```python
from build123d import *

# Parameters (mm, degrees)
SKETCH_1_R          = 12.5
SKETCH_1_R_2        = 10
EXTRUDE_1_DEPTH     = 120
SKETCH_2_R          = 3.5
CUT_EXTRUDE_1_DEPTH = 12.5
SWEEP_3_PROFILE_R   = 3.5


with BuildPart() as part:
    # 草图1 → 凸台-拉伸1 (new body)
    with BuildSketch(Plane(origin=(0, 0, 0), x_dir=(1, 0, 0), z_dir=(0, 1, 0))):
        Circle(SKETCH_1_R)
        Circle(SKETCH_1_R_2, mode=Mode.SUBTRACT)
    extrude(amount=EXTRUDE_1_DEPTH)

    # 草图2 → 切除-拉伸1 (cut, symmetric)
    with BuildSketch(Plane(origin=(0, 0, 0), x_dir=(0, 0, -1), z_dir=(1, 0, 0))):
        with Locations((0, 60)):
            Circle(SKETCH_2_R)
    extrude(amount=CUT_EXTRUDE_1_DEPTH, both=True, mode=Mode.SUBTRACT)

    # 切除-扫描3: sweep along a path in 草图10
    with BuildLine(Plane(origin=(0, 0, 0), x_dir=(0.342020143, 0, -0.939692621), z_dir=(0.939692621, 0, 0.342020143))) as sweep_3_path:
        Line((42.494333557, 116.01263537), (-37.5, 60))
        Line((-37.5, 60), (79.181849156, -21.701510351))
    # 切除-扫描3 profile (on start of the path) → 切除-扫描3 (sweep, cut)
    with BuildSketch(Plane(origin=(14.533918054, 116.01263537, -39.931611668), x_dir=(0, 0.801864671, 0.59750569), z_dir=(-0.2801665, -0.573576436, 0.769751131))):
        Circle(SWEEP_3_PROFILE_R)
    sweep(path=sweep_3_path.line, transition=Transition.RIGHT, mode=Mode.SUBTRACT)


solid = part.part
```
Geometry check sheet. Reference: the model listing, model coordinates, mm. Give positions to 0.01 mm unless a question says otherwise; leave off trailing zeros. Loops run counter-clockwise (first coordinate to the right, second up) from the corner with the lowest first, then second, coordinate; pieces in that order, holes last. Notation, with made-up numbers: M -12.75,74.25 L -4.75,74.25 A28 cw -4.75,101.25 Z; hole C -6,-5.75 d6. An arc over 180 degrees is marked long. Write item = value, one per line.
(1) Release check for a two-part mould opening along X. For faces 1 (the face through (1.314, 91.924, -11.921)), 2 (the face through (-0.1, 120, -10.2)), 3 (the face through (11.923, 59.16, -3.755)) record: released by +X, released by -X, zero draft, split by the parting line, or undercut.
Answer below:
face_1 = undercut
face_2 = zero draft
face_3 = split by the parting line
(2) Sectioned sample at C-C, the plane z = 5.75. Record the cut outline in (x, y).
Answer below:
outline = M -11.1,0 L -8.18,0 L -8.18,120 L -11.1,120 Z; M 8.18,0 L 11.1,0 L 11.1,120 L 8.18,120 Z
(3) Sectioned sample at A-A, the plane y = 60. Record the cut outline in (x, z).
Answer below:
outline = M -12,-3.5 A12.5 ccw 12,-3.5 L 9.37,-3.5 A10 cw -9.37,-3.5 Z; M -12,3.5 L -9.37,3.5 A10 cw 9.37,3.5 L 12,3.5 A12.5 ccw Z
(4) Gauge pin test, flat ends, axial feed: pin 1 Ø3 at (x, y) = (-4, 45) entering from +Z; pin 2 Ø12 at (y, z) = (102.5, -7) entering from -X; pin 3 Ø6 at (x, y) = (7, 106.5) entering from -Z. Record the tip position at first contact, or that the pin passes through.
Answer below:
pin_1 = 11.64
pin_2 = -12.46
pin_3 = -11.84
(5) Sectioned sample at B-B, the plane z = 0. Record the cut outline in (x, y), plus the area to 3 significant figures.
Answer below:
outline = M -12.5,0 L -10,0 L -10,56.5 L -12.5,56.5 Z; M -12.5,63.5 L -10,63.5 L -10,120 L -12.5,120 Z; M 10,0 L 12.5,0 L 12.5,56.5 L 10,56.5 Z; M 10,63.5 L 12.5,63.5 L 12.5,120 L 10,120 Z
area = 565 mm2
(6) Material ranges on line 1 (Y direction, x = 10.5, z = 0); line 2 (Z direction, x = -0.25, y = 102), recorded low to high. Write a range as [from, to].
Answer below:
line_1 = [0, 56.5], [63.5, 120]
line_2 = [-12.5, -10], [10, 12.5]
